```python
from build123d import *

# Parameters (mm, degrees)
BOSS_EXTRUDE1_DEPTH = 1.5
BOSS_EXTRUDE2_DEPTH = 5


with BuildPart() as part:
    # Sketch1 → Boss-Extrude1 (new body)
    with BuildSketch(Plane(origin=(0, 0, 0), x_dir=(1, 0, 0), z_dir=(0, 1, 0))):
        with BuildLine():
            Line((-25.910177173, 10.614269588), (-25.910177173, -10.614269588))
            ThreePointArc((-25.910177173, -10.614269588), (-22.603967361, -16.524547181), (-17.975471458, -21.468172392))
            Line((-17.975471458, -21.468172392), (17.975471458, -21.468172392))
            ThreePointArc((17.975471458, -21.468172392), (22.588149859, -16.546162273), (25.889822827, -10.663820796))
            Line((25.889822827, -10.663820796), (25.889822827, 10.663820796))
            ThreePointArc((25.889822827, 10.663820796), (22.650459328, 16.460762201), (18.137065113, 21.331827608))
            Line((18.137065113, 21.331827608), (-18.137065113, 21.331827608))
            ThreePointArc((-18.137065113, 21.331827608), (-22.666195109, 16.439087544), (-25.910177173, 10.614269588))
        make_face()
    extrude(amount=BOSS_EXTRUDE1_DEPTH)

    # Sketch2 → Boss-Extrude2 (add)
    with BuildSketch(Plane(origin=(0, 1.5, 0), x_dir=(1, 0, 0), z_dir=(0, 1, 0))):
        with BuildLine():
            Line((-17.283724515, 19.613012201), (-16.290407014, 18.48903696))
            ThreePointArc((-16.290407014, 18.48903696), (-19.977953658, 14.409984138), (-22.667306708, 9.613730147))
            Line((-22.667306708, 9.613730147), (-24.049459557, 10.196528143))
            ThreePointArc((-24.049459557, 10.196528143), (-21.196121564, 15.285236646), (-17.283724515, 19.613012201))
        make_face()
        with BuildLine():
            Line((17.283724515, 19.613012201), (16.290407014, 18.48903696))
            ThreePointArc((16.290407014, 18.48903696), (19.963841864, 14.42960445), (22.648482765, 9.658250436))
            Line((22.648482765, 9.658250436), (24.029487812, 10.243763084))
            ThreePointArc((24.029487812, 10.243763084), (21.181149295, 15.306053319), (17.283724515, 19.613012201))
        make_face()
        with BuildLine():
            Line((22.648482765, -9.546564422), (24.029487812, -10.13207707))
            ThreePointArc((24.029487812, -10.13207707), (21.121707142, -15.276589528), (17.131154209, -19.635108099))
            Line((17.131154209, -19.635108099), (16.146605116, -18.503444243))
            ThreePointArc((16.146605116, -18.503444243), (19.907815927, -14.395415244), (22.648482765, -9.546564422))
        make_face()
        with BuildLine():
            Line((-24.049459557, -10.08484213), (-22.667306708, -9.502044133))
            ThreePointArc((-22.667306708, -9.502044133), (-19.922003884, -14.375849937), (-16.146605116, -18.503444243))
            Line((-16.146605116, -18.503444243), (-17.131154209, -19.635108099))
            ThreePointArc((-17.131154209, -19.635108099), (-21.136760219, -15.255831214), (-24.049459557, -10.08484213))
        make_face()
    extrude(amount=BOSS_EXTRUDE2_DEPTH)


solid = part.part
```
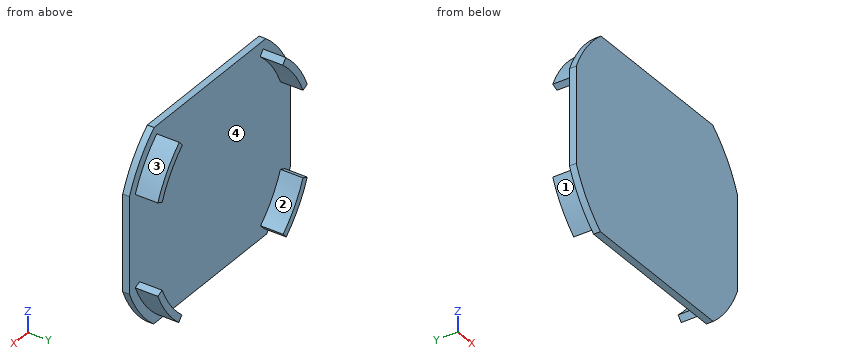
The listing builds one solid part. Answer for the finished solid, in the listing's coordinates (mm). Face numbers are marked on the shaded views. Give positions to 0.01 mm unless a question says otherwise; leave off trailing zeros. Order: outer loops, then holes, each group sorted by start corner. A loop starts at its lowest first (then second) coordinate and runs counter-clockwise, first axis right, second up. Notation, with made-up numbers: (-28.75, 22) -> (-21.75, 22) arc R17 ccw to (-21.75, 41) -> close; hole circle Ø3 at (19.5, 63.25). An arc over 180 degrees is marked (long way). One line per item, written item: value.
1) Find section A-A, the plane y = 4. Determine the outline of the cut face in (x, z), plus the area to 3 significant figures.
Reported:
outline: (-24.05, -10.2) arc R26.1 ccw to (-17.28, -19.61) -> (-16.29, -18.49) arc R24.6 cw to (-22.67, -9.61) -> close; (-24.05, 10.08) -> (-22.67, 9.5) arc R24.6 cw to (-16.15, 18.5) -> (-17.13, 19.64) arc R26.1 ccw to start; (16.15, 18.5) arc R24.6 cw to (22.65, 9.55) -> (24.03, 10.13) arc R26.1 ccw to (17.13, 19.64) -> close; (16.29, -18.49) -> (17.28, -19.61) arc R26.1 ccw to (24.03, -10.24) -> (22.65, -9.66) arc R24.6 cw to start
area: 68.6 mm^2
2) Find section D-D, the plane x = 19. Determine the outline of the cut face in (y, z), plus the area to 3 significant figures.
Reported:
outline: (0, -20.57) -> (1.5, -20.57) -> (1.5, -17.95) -> (6.5, -17.95) -> (6.5, -15.68) -> (1.5, -15.68) -> (1.5, 15.57) -> (6.5, 15.57) -> (6.5, 17.84) -> (1.5, 17.84) -> (1.5, 20.57) -> (0, 20.57) -> close
area: 84.4 mm^2
3) Flat-ended cylindrical pins translate along their axes: P1, Ø21.5, axis at x = -8.5, z = 9, coming from the +Y side; P2, Ø3, axis at x = 2, y = 3.5, coming from the -Z side; P3, Ø1, axis at x = -3.5, z = -11.5, coming from the -Y side. Find the tip coordinate at first contact, or state that the pin passes through.
Reported:
P1: stops at y = 1.5
P2: passes through
P3: stops at y = 0
4) Find section B-B, the plane x = -11.5. Determine the outline of the cut face in (y, z).
Reported:
outline: (0, -21.33) -> (1.5, -21.33) -> (1.5, 21.47) -> (0, 21.47) -> close
5) Find section C-C, the plane z = 6. Determine the outline of the cut face in (x, y).
Reported:
outline: (-25.91, 0) -> (25.89, 0) -> (25.89, 1.5) -> (-25.91, 1.5) -> close
6) Find the intervals of material crossed by line 1 (Y direction, x = 3, z = -17.5); line 2 (X direction, y = 4, z = -18); line 3 (X direction, y = 3, z = -15), in increasing order.
Reported:
line 1: y = 0 to 1.5
line 2: x = -18.95 to -16.83, 16.83 to 18.95
line 3: x = -21.4 to -19.54, 19.54 to 21.4
7) Determine the mould class of the marked faces 1, 2, 3 and 4 for opening direction X: pulls with the +X half, pulls with the -X half, needs draft (parallel to the pull), parting line crosses it, or undercut.
Reported:
face 1: pulls with the -X half
face 2: undercut
face 3: pulls with the +X half
face 4: undercut
